Input: dimensioned drawing with shaded views. Units: mm. Origin: part minimum x, y, z. A direction names the side the tool comes from. Coordinates: 2 decimals unless noted, no trailing zeros. Loops run counter-clockwise (first coordinate to the right, second up) from the corner with the lowest first, then second, coordinate; pieces in that order, holes last. Notation, with made-up numbers: (39.25, 73) -> (46.25, 73) arc R16 ccw to (46.25, 103) -> close; hole circle Ø5 at (19, 52). An arc over 180 degrees is marked (long way). Answer as CSV lines item,"result".
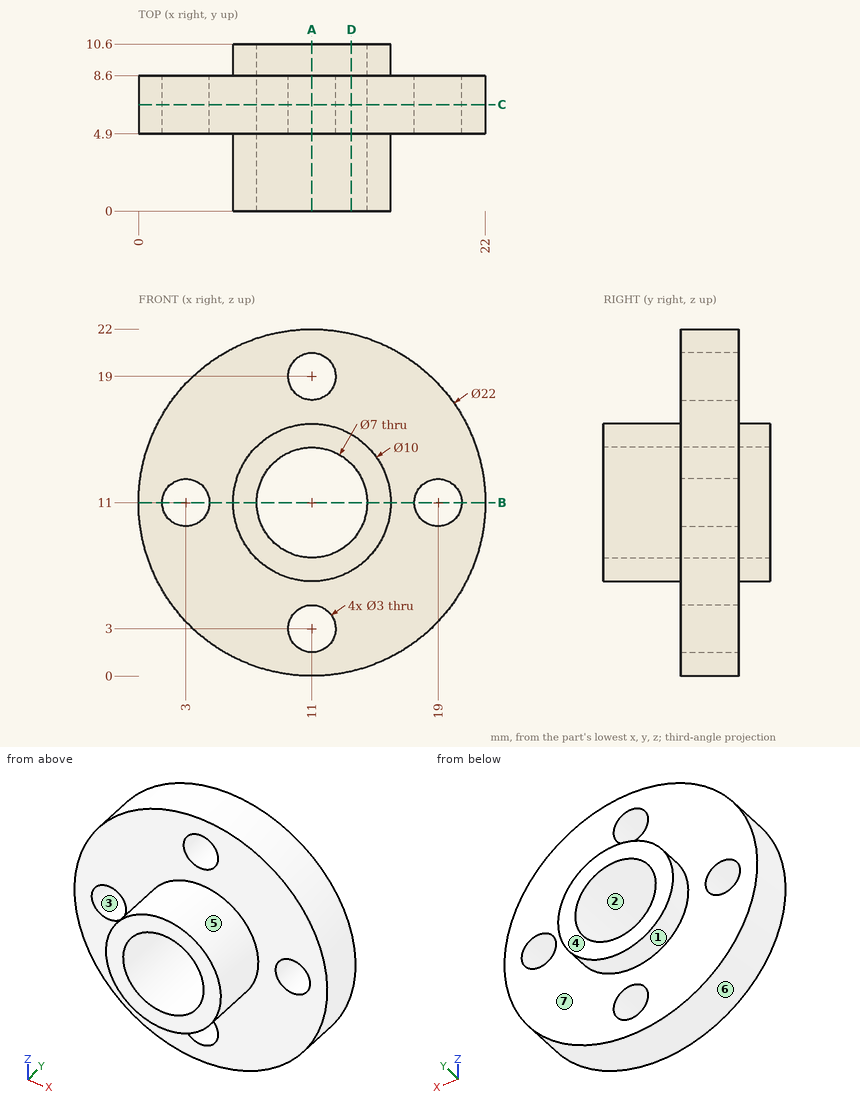
(1) Cut plane D-D (x = 13.5). Return the cut outline in (y, z), then the cut area to 3 significant figures.
Computed values:
outline,"(0, 6.67) -> (4.9, 6.67) -> (4.9, 0.29) -> (8.6, 0.29) -> (8.6, 6.67) -> (10.6, 6.67) -> (10.6, 8.55) -> (0, 8.55) -> close; (0, 13.45) -> (10.6, 13.45) -> (10.6, 15.33) -> (8.6, 15.33) -> (8.6, 21.71) -> (4.9, 21.71) -> (4.9, 15.33) -> (0, 15.33) -> close"
area,"87.1 mm^2"
(2) Material intervals for L1, parallel to X at y = 7.3, z = 11; L2, parallel to X at y = 7.25, z = 12.25; L3, parallel to Y at x = 14, z = 18.5, sorted ascending. Write a range as [from, to].
Computed values:
L1,"[0, 1.5], [4.5, 7.5], [14.5, 17.5], [20.5, 22]"
L2,"[0.07, 2.17], [3.83, 7.73], [14.27, 18.17], [19.83, 21.93]"
L3,"[4.9, 8.6]"
(3) Cut plane A-A (x = 11). Return the cut outline in (y, z), then the cut area to 3 significant figures.
Computed values:
outline,"(0, 6) -> (4.9, 6) -> (4.9, 4.5) -> (8.6, 4.5) -> (8.6, 6) -> (10.6, 6) -> (10.6, 7.5) -> (0, 7.5) -> close; (0, 14.5) -> (10.6, 14.5) -> (10.6, 16) -> (8.6, 16) -> (8.6, 17.5) -> (4.9, 17.5) -> (4.9, 16) -> (0, 16) -> close; (4.9, 0) -> (8.6, 0) -> (8.6, 1.5) -> (4.9, 1.5) -> close; (4.9, 20.5) -> (8.6, 20.5) -> (8.6, 22) -> (4.9, 22) -> close"
area,"54.0 mm^2"
(4) Draft query along Z for the marked faces 1, 2, 3 and 4. Return one class per face: released by +Z, released by -Z, zero draft, split by the parting line, or undercut.
Computed values:
face 1,"split by the parting line"
face 2,"undercut"
face 3,"undercut"
face 4,"zero draft"
(5) Pin query (flat end, axial travel): pin 1 Ø10 at (x, z) = (2.5, 12.5) entering from +Y; pin 2 Ø3.5 at (x, z) = (19, 11) entering from +Y; pin 3 Ø1 at (x, y) = (15, 9.5) entering from +Z; pin 4 Ø4 at (x, z) = (3, 16) entering from -Y. Return the tip coordinate at first contact, or that it passes through.
Computed values:
pin 1,"y = 10.6"
pin 2,"y = 8.6"
pin 3,"z = 14.57"
pin 4,"y = 4.9"
(6) Cut plane B-B (z = 11). Return the cut outline in (x, y).
Computed values:
outline,"(0, 4.9) -> (1.5, 4.9) -> (1.5, 8.6) -> (0, 8.6) -> close; (4.5, 4.9) -> (6, 4.9) -> (6, 0) -> (7.5, 0) -> (7.5, 10.6) -> (6, 10.6) -> (6, 8.6) -> (4.5, 8.6) -> close; (14.5, 0) -> (16, 0) -> (16, 4.9) -> (17.5, 4.9) -> (17.5, 8.6) -> (16, 8.6) -> (16, 10.6) -> (14.5, 10.6) -> close; (20.5, 4.9) -> (22, 4.9) -> (22, 8.6) -> (20.5, 8.6) -> close"
(7) Access query for the marked faces 5, 6 and 7. Directions: +Z, -Z, +X, -X, +Y, -Y. A direction counts if a zero-diameter tool reaches every point of the face in a straight line with its end or side. Return the directions, or none.
Computed values:
face 5,"-Y"
face 6,"+Y, -Y"
face 7,"+Y"
(8) Cut plane C-C (y = 6.75). Return the cut outline in (x, z).
Computed values:
outline,"circle Ø22 at (11, 11); hole circle Ø3 at (3, 11); hole circle Ø7 at (11, 11); hole circle Ø3 at (11, 3); hole circle Ø3 at (11, 19); hole circle Ø3 at (19, 11)"
